from build123d import *

# Parameters (mm, degrees)
SKETCH2_R           = 4.1
SKETCH2_R_2         = 1.455
BOSS_EXTRUDE2_DEPTH = 10


with BuildPart() as part:
    # Sketch2 → Boss-Extrude2 (new body)
    with BuildSketch(Plane(origin=(0, 0, 0), x_dir=(-1, 0, 0), z_dir=(0, 1, 0))):
        with BuildLine():
            Line((5.045766375, -9.830704028), (36.565058692, 6.347077836))
            ThreePointArc((36.565058692, 6.347077836), (39.606684002, 6.595535729), (41.933124145, 4.620468108))
            Line((41.933124145, 4.620468108), (220.6412412, -343.557880956))
            Line((220.6412412, -343.557880956), (240.302649257, -333.466348206))
            Line((240.302649257, -333.466348206), (61.594532201, 14.712000858))
            ThreePointArc((61.594532201, 14.712000858), (46.373607726, 27.634041934), (26.473525942, 26.008485892))
            Line((26.473525942, 26.008485892), (-5.045766375, 9.830704028))
            ThreePointArc((-5.045766375, 9.830704028), (-9.830704028, -5.045766375), (5.045766375, -9.830704028))
        make_face()
        Circle(SKETCH2_R, mode=Mode.SUBTRACT)
        with Locations((-3.653043529, 7.117251785)):
            Circle(SKETCH2_R_2, mode=Mode.SUBTRACT)
        with Locations((7.117251785, 3.653043529)):
            Circle(SKETCH2_R_2, mode=Mode.SUBTRACT)
        with Locations((-7.117251785, -3.653043529)):
            Circle(SKETCH2_R_2, mode=Mode.SUBTRACT)
        with Locations((3.653043529, -7.117251785)):
            Circle(SKETCH2_R_2, mode=Mode.SUBTRACT)
    extrude(amount=BOSS_EXTRUDE2_DEPTH)


solid = part.part
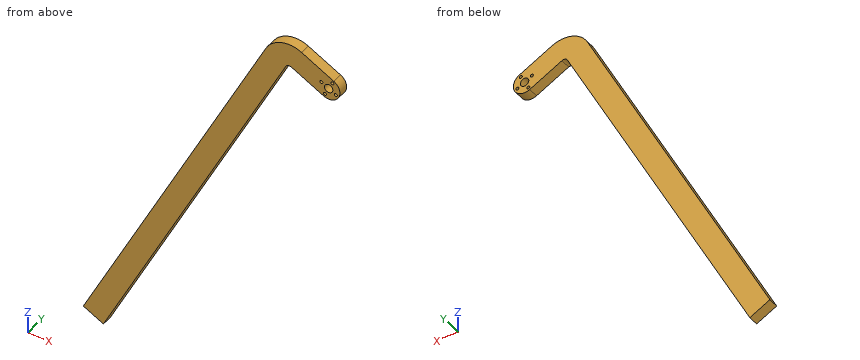
Work out the finished part from the listing and answer in its coordinate system (mm). Round coordinates to 2 decimals unless told otherwise and drop trailing zeros. Loops run counter-clockwise (first coordinate to the right, second up) from the corner with the lowest first, then second, coordinate; pieces in that order, holes last. Notation, with made-up numbers: (8.25, -27.75) - (18.25, -27.75) arc R21 cw to (18.25, 1.25) - close; hole circle Ø9 at (7, 59.25). An arc over 180 degrees is marked (long way). Use one line per item in the form item = value. Start each with the question number.
(1) Find section C-C on z = -154.5. Determine the outline of the cut face in (x, y), and give its area (3 significant figures).
(2) Find section B-B on x = -105. Determine the outline of the cut face in (y, z).
(3) Flat-ended cylindrical pins translate along their axes: P1, Ø2.5, axis at x = -3.65, z = -7.12, coming from the -Y side; P2, Ø3, axis at x = -156, y = 8, coming from the -Z side; P3, Ø1, axis at x = -157, y = 2, coming from the +Z side; P4, Ø3, axis at y = 4, z = -122.5, coming from the +X side. Find the tip coordinate at first contact, or state that the pin passes through.
(4) Find section A-A on y = 4.5. Determine the outline of the cut face in (x, z) (3 decimals).
(5) Consider line 1 (Z direction, x = -3.5, y = 4); line 2 (X direction, y = 0.5, z = -228.5); line 3 (Z direction, x = -45.5, y = 9). Determine where each line is inside the solid, lowest interval first.
Answer list:
q1.outline = (-148.45, 0) - (-123.6, 0) - (-123.6, 10) - (-148.45, 10) - close
q1.area = 248 mm^2
q2.outline = (0, -118.25) - (10, -118.25) - (10, -69.86) - (0, -69.86) - close
q3.P1 = through
q3.P2 = -220.54
q3.P3 = -170.19
q3.P4 = -106.41
q4.outline = (-240.303, -333.466) - (-220.641, -343.558) - (-41.933, 4.62) arc R3.987 cw to (-36.565, 6.347) - (-5.046, -9.831) arc R11.05 ccw to (5.046, 9.831) - (-26.474, 26.008) arc R26.087 ccw to (-61.595, 14.712) - close; hole circle Ø2.91 at (-7.117, 3.653); hole circle Ø2.91 at (-3.653, -7.117); hole circle Ø8.2 at (0, 0); hole circle Ø2.91 at (3.653, 7.117); hole circle Ø2.91 at (7.117, -3.653)
q5.line_1 = -10.48 to -8.56, -5.67 to -2.14, 2.14 to 14.22
q5.line_2 = -186.43 to -161.59
q5.line_3 = -2.33 to 27.9
